Read the model definition and answer for the solid it produces. Units are mm, in the model's axes. Give positions to 0.01 mm unless a question says otherwise; leave off trailing zeros. Order: outer loops, then holes, each group sorted by start corner. A loop starts at its lowest first (then second) coordinate and runs counter-clockwise, first axis right, second up. Notation, with made-up numbers: (-18.75, 13.5) -> (2.25, 13.5) arc R14 ccw to (2.25, 17.5) -> close; hole circle Ø7 at (20.25, -24.5). An arc over 180 degrees is marked (long way). Answer as CSV lines item,"result". Start each with the question number.
1) The mould has two halves that part along X. Classify faces 1 (the face through (6.284, 1.268, -8.615)), 2 (the face through (38.025, 1.479, -29.415)), 3 (the face through (0, 1, -9)), 4 (the face through (22, 0, -18)): +X half, -X half, draft (parallel to the pull), parting line (faces both ways), or undercut.
2) Find section D-D (z = -23.5). Determine the outline of the cut face in (x, y), and give its area (3 significant figures).
3) Find section C-C (x = 37.5). Determine the outline of the cut face in (y, z).
4) Find section B-B (y = 1.05). Determine the outline of the cut face in (x, z).
5) Find section A-A (x = 22.5). Determine the outline of the cut face in (y, z), and give its area (3 significant figures).
6) Straight lines are drawn through the part: L1, parallel to Z at x = 22.5, y = 1.9; L2, parallel to X at y = 1.65, z = -7.5; L3, parallel to X at y = 2.4, z = -8.5. For each, find the intervals that lie inside material, in ascending order. Write a range as from..to.
7) Flat-ended cylindrical pins translate along their axes: pin 1 Ø2.5 at (x, z) = (22.5, -38.5) entering from -Y; pin 2 Ø6 at (x, z) = (15.5, -17) entering from +Y; pin 3 Ø1.5 at (y, z) = (2, -35.5) entering from +X. Find the tip coordinate at first contact, or state that the pin passes through.
```python
from build123d import *

# Parameters (mm, degrees)
EXTRUDE_1_DEPTH     = 3
SKETCH_2_R          = 1.65
CUT_EXTRUDE_1_DEPTH = 3
FILLET_1_R          = 5
CUT_EXTRUDE_2_DEPTH = 0.5


with BuildPart() as part:
    # ｽｹｯﾁ1 → ﾎﾞｽ - 押し出し1 (new body)
    with BuildSketch(Plane(origin=(0, 0, 0), x_dir=(1, 0, 0), z_dir=(0, 1, 0))):
        Polygon((0, 0), (45, 0), (45, 15), (30, 46), (15, 46), (0, 15), align=None)
    extrude(amount=EXTRUDE_1_DEPTH)

    # ｽｹｯﾁ2 → ｶｯﾄ - 押し出し1 (cut)
    with BuildSketch(Plane(origin=(0, 3, 0), x_dir=(1, 0, 0), z_dir=(0, 1, 0))):
        with Locations((7.5, 7.5)):
            Circle(SKETCH_2_R)
        with Locations((22.5, 38.5)):
            Circle(SKETCH_2_R)
        with Locations((22.5, 23.5)):
            Circle(SKETCH_2_R)
        with Locations((37.5, 7.5)):
            Circle(SKETCH_2_R)
    extrude(amount=-CUT_EXTRUDE_1_DEPTH, mode=Mode.SUBTRACT)

    # ﾌｨﾚｯﾄ1
    fillet_1_edges = [part.edges().sort_by_distance(p)[0] for p in [
        (0, 1.5, -15),
        (15, 1.5, -46),
        (30, 1.5, -46),
        (45, 1.5, -15),
        (45, 1.5, 0),
        (0, 1.5, 0),
    ]]
    fillet(fillet_1_edges, radius=FILLET_1_R)

    # ｽｹｯﾁ3 → ｶｯﾄ - 押し出し2 (cut)
    with BuildSketch(Plane(origin=(0, 3, 0), x_dir=(1, 0, 0), z_dir=(0, 1, 0))):
        Polygon((0, 0), (45, 0), (45, 15.05), (30.05, 15.05), (30.05, 46), (14.95, 46), (14.95, 15.05), (0, 15.05), align=None)
    extrude(amount=-CUT_EXTRUDE_2_DEPTH, mode=Mode.SUBTRACT)


solid = part.part
```
Findings below:
1,face 1,"undercut"
1,face 2,"+X half"
1,face 3,"-X half"
1,face 4,"draft"
2,outline,"(4.11, 0) -> (20.85, 0) -> (20.85, 2.5) -> (14.95, 2.5) -> (14.95, 3) -> (4.11, 3) -> close; (24.15, 0) -> (40.89, 0) -> (40.89, 3) -> (30.05, 3) -> (30.05, 2.5) -> (24.15, 2.5) -> close"
2,area,"94.5 mm²"
3,outline,"(0, -30.5) -> (3, -30.5) -> (3, -15.05) -> (2.5, -15.05) -> (2.5, -9.15) -> (0, -9.15) -> close; (0, -5.85) -> (2.5, -5.85) -> (2.5, 0) -> (0, 0) -> close"
4,outline,"(0, -13.85) arc R5 ccw to (0.5, -16.03) -> (13.63, -43.18) arc R5 ccw to (18.14, -46) -> (26.86, -46) arc R5 ccw to (31.37, -43.18) -> (44.5, -16.03) arc R5 ccw to (45, -13.85) -> (45, -5) arc R5 ccw to (40, 0) -> (5, 0) arc R5 ccw to (0, -5) -> close; hole circle Ø3.3 at (7.5, -7.5); hole circle Ø3.3 at (22.5, -38.5); hole circle Ø3.3 at (22.5, -23.5); hole circle Ø3.3 at (37.5, -7.5)"
5,outline,"(0, -46) -> (2.5, -46) -> (2.5, -40.15) -> (0, -40.15) -> close; (0, -36.85) -> (2.5, -36.85) -> (2.5, -25.15) -> (0, -25.15) -> close; (0, -21.85) -> (2.5, -21.85) -> (2.5, 0) -> (0, 0) -> close"
5,area,"98.5 mm²"
6,L1,"-46..-40.15, -36.85..-25.15, -21.85..0"
6,L2,"0..5.85, 9.15..35.85, 39.15..45"
6,L3,"0..6.19, 8.81..36.19, 38.81..45"
7,pin 1,"through"
7,pin 2,"y = 3"
7,pin 3,"x = 35.44"
